Work out the finished part from the listing and answer in its coordinate system (mm). Face numbers are marked on the shaded views. A direction names the side the tool comes from. Round coordinates to 2 decimals unless told otherwise and drop trailing zeros. Loops run counter-clockwise (first coordinate to the right, second up) from the corner with the lowest first, then second, coordinate; pieces in that order, holes last. Notation, with made-up numbers: (12.5, 43.25) - (29.5, 43.25) arc R34 cw to (29.5, 73.25) - close; hole circle Ø11 at (69.25, 11.5). An arc over 180 degrees is marked (long way). Return JSON: item names as keys, results as strings.
from build123d import *

# Parameters (mm, degrees)
BOSS_EXTRUDE1_DEPTH = 6.2
BOSS_EXTRUDE2_DEPTH = 21
CHAMFER1_SIZE       = 5
CHAMFER1_SIZE2      = 28.356409098
CUT_EXTRUDE1_REACH  = 74.109
CHAMFER2_SIZE       = 1
CHAMFER2_SIZE2      = 9.514364454
CHAMFER3_SIZE       = 2
CUT_EXTRUDE2_REACH  = 79.092
CUT_EXTRUDE3_START  = -3.468867
CUT_EXTRUDE3_DEPTH  = 3.468867
BOSS_EXTRUDE3_DEPTH = 6.2
CUT_EXTRUDE4_REACH  = 79.092
CUT_EXTRUDE5_DEPTH  = 73.108598655
CUT_EXTRUDE6_REACH  = 74.109


with BuildPart() as part:
    # Sketch1 → Boss-Extrude1 (new body)
    with BuildSketch(Plane.XY):
        with BuildLine():
            Line((-28.3, 0), (0, 0))
            Line((0, 0), (0, 10))
            Line((0, 10), (-7.1, 10))
            ThreePointArc((-7.1, 10), (-14.171067812, 12.928932188), (-17.1, 20))
            Line((-17.1, 20), (-17.1, 51))
            Line((-17.1, 51), (-20.1, 51))
            Line((-20.1, 51), (-20.1, 6))
            Line((-20.1, 6), (-24.3, 6))
            Line((-24.3, 6), (-24.3, 50))
            Line((-24.3, 50), (-28.3, 50))
            Line((-28.3, 50), (-28.3, 0))
        make_face()
    extrude(amount=BOSS_EXTRUDE1_DEPTH)

    # Sketch2 → Boss-Extrude2 (add)
    with BuildSketch(Plane.XZ):
        Polygon((0, 6.2), (0, 10.4), (11, 10.4), (11, 42.4), (-24.1, 42.4), (-24.1, 10.4), (-13.1, 10.4), (-13.1, 6.2), align=None)
    extrude(amount=-BOSS_EXTRUDE2_DEPTH)

    # Chamfer1
    chamfer1_edges = [part.edges().sort_by_distance(p)[0] for p in [
        (-6.55, 0, 42.4),
    ]]
    chamfer1_side = [part.faces().sort_by_distance(p)[0] for p in [
        (-6.55, 10.5, 42.4),
    ]]
    chamfer(chamfer1_edges, length=CHAMFER1_SIZE, length2=CHAMFER1_SIZE2, reference=chamfer1_side[0])

    # Sketch3 → Cut-Extrude1 (cut, up to next)
    with BuildSketch(Plane(origin=(0, 0, 0), x_dir=(0, 0, -1), z_dir=(1, 0, 0)), mode=Mode.PRIVATE) as cut_extrude1_sk1:
        Polygon((-6.2, 10), (-7.6, 10), (-10.4, 21), (-6.2, 21), align=None)
    cut_extrude1_tool1 = extrude(cut_extrude1_sk1.sketch, amount=-CUT_EXTRUDE1_REACH, mode=Mode.PRIVATE) & part.part
    add(cut_extrude1_tool1.solids().sort_by_distance((0, 16.416667, 7.716667))[0], mode=Mode.SUBTRACT)

    # Chamfer2
    chamfer2_edges = [part.edges().sort_by_distance(p)[0] for p in [
        (11, 10.5, 10.4),
    ]]
    chamfer2_side = [part.faces().sort_by_distance(p)[0] for p in [
        (11, 11.541747932, 25.62778603),
    ]]
    chamfer(chamfer2_edges, length=CHAMFER2_SIZE, length2=CHAMFER2_SIZE2, reference=chamfer2_side[0])

    # Chamfer3
    chamfer3_edges = [part.edges().sort_by_distance(p)[0] for p in [
        (-24.1, 10.5, 10.4),
    ]]
    chamfer(chamfer3_edges, length=CHAMFER3_SIZE)

    # Sketch5 → Cut-Extrude2 (cut, up to next)
    with BuildSketch(Plane(origin=(11, 0, 0), x_dir=(0, 0, -1), z_dir=(1, 0, 0)), mode=Mode.PRIVATE) as cut_extrude2_sk1:
        Polygon((-42.4, 17.8), (-13.86886709, 5), (-10.966215349, -4.108657177), (-44.036924755, 0.937700744), align=None)
    cut_extrude2_tool1 = extrude(cut_extrude2_sk1.sketch, amount=-CUT_EXTRUDE2_REACH, mode=Mode.PRIVATE) & part.part
    add(cut_extrude2_tool1.solids().sort_by_distance((11, 5.258773, 29.627692))[0], mode=Mode.SUBTRACT)

    # Sketch6 → Cut-Extrude3 (cut)
    with BuildSketch(Plane(origin=(0, 0, 10.4), x_dir=(-1, 0, 0), z_dir=(0, 0, -1)).offset(CUT_EXTRUDE3_START)):
        Polygon((13.1, 0), (24.1, 5), (37.198342989, 5), (28.62602328, -4.522208447), (-13.825974113, -5.629287686), (-20.705007466, 5), (-11, 5), (0, 0), align=None)
    extrude(amount=CUT_EXTRUDE3_DEPTH, mode=Mode.SUBTRACT)

    # Sketch7 → Boss-Extrude3 (add)
    with BuildSketch(Plane.XY.offset(6.2)):
        with BuildLine():
            Line((-16.7, 50.6), (-15.7, 50.5))
            ThreePointArc((-15.7, 50.5), (-15.462165524, 50.365875857), (-15.4, 50.1))
            ThreePointArc((-15.4, 50.1), (-15.462165524, 49.834124143), (-15.7, 49.7))
            Line((-15.7, 49.7), (-16.7, 49.6))
            ThreePointArc((-16.7, 49.6), (-16.971392676, 49.471392676), (-17.1, 49.2))
            Line((-17.1, 49.2), (-17.1, 48.7))
            ThreePointArc((-17.1, 48.7), (-16.971392676, 48.428607324), (-16.7, 48.3))
            Line((-16.7, 48.3), (-15.7, 48.2))
            ThreePointArc((-15.7, 48.2), (-15.462165524, 48.065875857), (-15.4, 47.8))
            ThreePointArc((-15.4, 47.8), (-15.462165524, 47.534124143), (-15.7, 47.4))
            Line((-15.7, 47.4), (-16.7, 47.3))
            ThreePointArc((-16.7, 47.3), (-16.971392676, 47.171392676), (-17.1, 46.9))
            Line((-17.1, 46.9), (-17.1, 46.4))
            ThreePointArc((-17.1, 46.4), (-16.971392676, 46.128607324), (-16.7, 46))
            Line((-16.7, 46), (-15.7, 45.9))
            ThreePointArc((-15.7, 45.9), (-15.462165524, 45.765875857), (-15.4, 45.5))
            ThreePointArc((-15.4, 45.5), (-15.462165524, 45.234124143), (-15.7, 45.1))
            Line((-15.7, 45.1), (-16.7, 45))
            ThreePointArc((-16.7, 45), (-16.971392676, 44.871392676), (-17.1, 44.6))
            Line((-17.1, 44.6), (-17.1, 44.1))
            ThreePointArc((-17.1, 44.1), (-16.971392676, 43.828607324), (-16.7, 43.7))
            Line((-16.7, 43.7), (-15.7, 43.6))
            ThreePointArc((-15.7, 43.6), (-15.462165524, 43.465875857), (-15.4, 43.2))
            ThreePointArc((-15.4, 43.2), (-15.462165524, 42.934124143), (-15.7, 42.8))
            Line((-15.7, 42.8), (-16.7, 42.7))
            ThreePointArc((-16.7, 42.7), (-16.971392676, 42.571392676), (-17.1, 42.3))
            Line((-17.1, 42.3), (-17.1, 41.8))
            ThreePointArc((-17.1, 41.8), (-16.971392676, 41.528607324), (-16.7, 41.4))
            Line((-16.7, 41.4), (-15.7, 41.3))
            ThreePointArc((-15.7, 41.3), (-15.462165524, 41.165875857), (-15.4, 40.9))
            ThreePointArc((-15.4, 40.9), (-15.462165524, 40.634124143), (-15.7, 40.5))
            Line((-15.7, 40.5), (-16.7, 40.4))
            ThreePointArc((-16.7, 40.4), (-16.971392676, 40.271392676), (-17.1, 40))
            Line((-17.1, 40), (-17.1, 39.5))
            ThreePointArc((-17.1, 39.5), (-16.971392676, 39.228607324), (-16.7, 39.1))
            Line((-16.7, 39.1), (-15.7, 39))
            ThreePointArc((-15.7, 39), (-15.462165524, 38.865875857), (-15.4, 38.6))
            ThreePointArc((-15.4, 38.6), (-15.462165524, 38.334124143), (-15.7, 38.2))
            Line((-15.7, 38.2), (-16.7, 38.1))
            ThreePointArc((-16.7, 38.1), (-16.971392676, 37.971392676), (-17.1, 37.7))
            Line((-17.1, 37.7), (-17.1, 37.2))
            ThreePointArc((-17.1, 37.2), (-16.971392676, 36.928607324), (-16.7, 36.8))
            Line((-16.7, 36.8), (-15.7, 36.7))
            ThreePointArc((-15.7, 36.7), (-15.462165524, 36.565875857), (-15.4, 36.3))
            ThreePointArc((-15.4, 36.3), (-15.462165524, 36.034124143), (-15.7, 35.9))
            Line((-15.7, 35.9), (-16.7, 35.8))
            ThreePointArc((-16.7, 35.8), (-16.971392676, 35.671392676), (-17.1, 35.4))
            Line((-17.1, 35.4), (-17.1, 34.9))
            ThreePointArc((-17.1, 34.9), (-16.971392676, 34.628607324), (-16.7, 34.5))
            Line((-16.7, 34.5), (-15.7, 34.4))
            ThreePointArc((-15.7, 34.4), (-15.462165524, 34.265875857), (-15.4, 34))
            ThreePointArc((-15.4, 34), (-15.462165524, 33.734124143), (-15.7, 33.6))
            Line((-15.7, 33.6), (-16.7, 33.5))
            ThreePointArc((-16.7, 33.5), (-16.971392676, 33.371392676), (-17.1, 33.1))
            Line((-17.1, 33.1), (-17.1, 32.6))
            ThreePointArc((-17.1, 32.6), (-16.971392676, 32.328607324), (-16.7, 32.2))
            Line((-16.7, 32.2), (-15.7, 32.1))
            ThreePointArc((-15.7, 32.1), (-15.462165524, 31.965875857), (-15.4, 31.7))
            ThreePointArc((-15.4, 31.7), (-15.462165524, 31.434124143), (-15.7, 31.3))
            Line((-15.7, 31.3), (-16.7, 31.2))
            ThreePointArc((-16.7, 31.2), (-16.971392676, 31.071392676), (-17.1, 30.8))
            Line((-17.1, 30.8), (-17.1, 30.3))
            ThreePointArc((-17.1, 30.3), (-16.971392676, 30.028607324), (-16.7, 29.9))
            Line((-16.7, 29.9), (-15.7, 29.8))
            ThreePointArc((-15.7, 29.8), (-15.462165524, 29.665875857), (-15.4, 29.4))
            ThreePointArc((-15.4, 29.4), (-15.462165524, 29.134124143), (-15.7, 29))
            Line((-15.7, 29), (-16.7, 28.9))
            ThreePointArc((-16.7, 28.9), (-16.971392676, 28.771392676), (-17.1, 28.5))
            Line((-17.1, 28.5), (-17.1, 28))
            ThreePointArc((-17.1, 28), (-16.971392676, 27.728607324), (-16.7, 27.6))
            Line((-16.7, 27.6), (-15.7, 27.5))
            ThreePointArc((-15.7, 27.5), (-15.462165524, 27.365875857), (-15.4, 27.1))
            ThreePointArc((-15.4, 27.1), (-15.462165524, 26.834124143), (-15.7, 26.7))
            Line((-15.7, 26.7), (-16.7, 26.6))
            ThreePointArc((-16.7, 26.6), (-16.971392676, 26.471392676), (-17.1, 26.2))
            Line((-17.1, 26.2), (-17.1, 25.7))
            ThreePointArc((-17.1, 25.7), (-16.971392676, 25.428607324), (-16.7, 25.3))
            Line((-16.7, 25.3), (-15.7, 25.2))
            ThreePointArc((-15.7, 25.2), (-15.462165524, 25.065875857), (-15.4, 24.8))
            ThreePointArc((-15.4, 24.8), (-15.462165524, 24.534124143), (-15.7, 24.4))
            Line((-15.7, 24.4), (-16.7, 24.3))
            ThreePointArc((-16.7, 24.3), (-16.971392676, 24.171392676), (-17.1, 23.9))
            Line((-17.1, 23.9), (-17.1, 23.4))
            ThreePointArc((-17.1, 23.4), (-16.971392676, 23.128607324), (-16.7, 23))
            Line((-16.7, 23), (-15.7, 22.9))
            ThreePointArc((-15.7, 22.9), (-15.462165524, 22.765875857), (-15.4, 22.5))
            ThreePointArc((-15.4, 22.5), (-15.462165524, 22.234124143), (-15.7, 22.1))
            Line((-15.7, 22.1), (-16.7, 22))
            ThreePointArc((-16.7, 22), (-16.971392676, 21.871392676), (-17.1, 21.6))
            Line((-17.1, 21.6), (-17.1, 21.1))
            ThreePointArc((-17.1, 21.1), (-16.971392676, 20.828607324), (-16.7, 20.7))
            Line((-16.7, 20.7), (-15.7, 20.6))
            ThreePointArc((-15.7, 20.6), (-15.462165524, 20.465875857), (-15.4, 20.2))
            ThreePointArc((-15.4, 20.2), (-15.462165524, 19.934124143), (-15.7, 19.8))
            Line((-15.7, 19.8), (-16.7, 19.7))
            ThreePointArc((-16.7, 19.7), (-16.971392676, 19.571392676), (-17.1, 19.3))
            Line((-17.1, 19.3), (-17.1, 18.8))
            Line((-17.1, 18.8), (-18.685, 49.2))
            Line((-18.685, 49.2), (-17.1, 51))
            ThreePointArc((-17.1, 51), (-16.971392676, 50.728607324), (-16.7, 50.6))
        make_face()
    extrude(amount=-BOSS_EXTRUDE3_DEPTH)

    # Sketch8 → Cut-Extrude4 (cut, up to next)
    with BuildSketch(Plane(origin=(11, 0, 0), x_dir=(0, 0, -1), z_dir=(1, 0, 0)), mode=Mode.PRIVATE) as cut_extrude4_sk1:
        Polygon((-35.4, 21), (-27.4, 17), (-19.4, 21), align=None)
    cut_extrude4_tool1 = extrude(cut_extrude4_sk1.sketch, amount=-CUT_EXTRUDE4_REACH, mode=Mode.PRIVATE) & part.part
    add(cut_extrude4_tool1.solids().sort_by_distance((11, 19.666667, 27.4))[0], mode=Mode.SUBTRACT)

    # Sketch10 → Cut-Extrude5 (cut, through all)
    with BuildSketch(Plane.XY.offset(42.4)):
        Polygon((-11.55, 21), (-6.55, 19), (-1.55, 21), align=None)
    extrude(amount=-CUT_EXTRUDE5_DEPTH, mode=Mode.SUBTRACT)

    # Sketch11 → Cut-Extrude6 (cut, up to next)
    with BuildSketch(Plane(origin=(0, 0, 0), x_dir=(-1, 0, 0), z_dir=(0, 0, -1)), mode=Mode.PRIVATE) as cut_extrude6_sk1:
        Polygon((24.3, 23.549969474), (24.6, 5.974018531), (19.8, 5.974018531), (20.1, 30.243837205), align=None)
    cut_extrude6_tool1 = extrude(cut_extrude6_sk1.sketch, amount=-CUT_EXTRUDE6_REACH, mode=Mode.PRIVATE) & part.part
    add(cut_extrude6_tool1.solids().sort_by_distance((-22.072028, 16.298165, 0))[0], mode=Mode.SUBTRACT)


solid = part.part
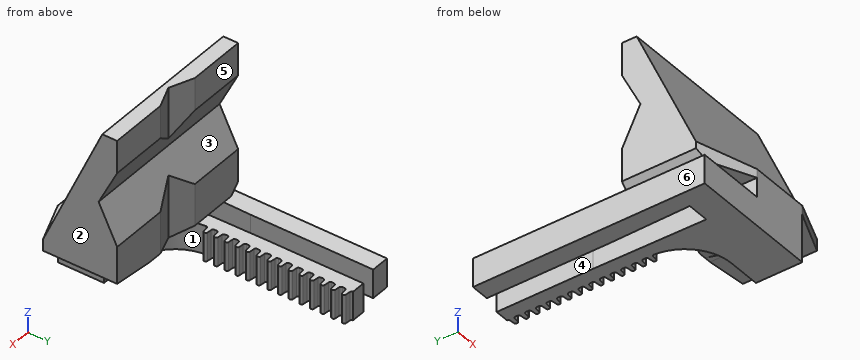
1) Find the intervals of material crossed by L1, parallel to X at y = 13.5, z = 32; L2, parallel to Z at x = -16, y = 32; L3, parallel to Y at x = -22, z = 2, in increasing order.
Verdict:
{"L1": "x = -24.1 to 11", "L2": "z = 0 to 6.2", "L3": "y = 0 to 5.97"}
2) Section A-A (y = 13) is taken. Give the vertices of the cut face in (x, z), and give its area (3 significant figures).
Verdict:
{"outline": "(-28.3, 0) - (-24.48, 0) - (-24.48, 6.2) - (-28.3, 6.2) - close; (-24.1, 12.4) - (-22.1, 10.4) - (-13.1, 10.4) - (-13.1, 8.36) - (0, 8.36) - (0, 10.4) - (1.49, 10.4) - (11, 11.4) - (11, 31.7) - (-24.1, 31.7) - close; (-19.89, 0) - (-14.24, 0) - (-14.24, 6.2) - (-19.89, 6.2) - close", "area": "826 mm2"}
3) Determine the mould class of the marked faces 1, 2 and 3 for opening direction Y: pulls with the +Y half, pulls with the -Y half, needs draft (parallel to the pull), parting line crosses it, or undercut.
Verdict:
{"face 1": "undercut", "face 2": "needs draft", "face 3": "pulls with the +Y half"}
4) Section C-C (x = -21) is taken. Give the vertices of the cut face in (y, z).
Verdict:
{"outline": "(0, 0) - (5.97, 0) - (5.97, 6.2) - (0, 6.2) - close; (3.59, 10.4) - (21, 10.4) - (21, 19.4) - (17, 27.4) - (21, 35.4) - (21, 42.4) - (17.8, 42.4) - (5, 13.87) - (3.59, 13.42) - close"}
5) Section B-B (z = 38) is taken. Give the vertices of the cut face in (x, y).
Verdict:
{"outline": "(-24.1, 15.83) - (11, 15.83) - (11, 21) - (-1.55, 21) - (-6.55, 19) - (-11.55, 21) - (-24.1, 21) - close"}
6) Section D-D (z = 17) is taken. Give the vertices of the cut face in (x, y), and give its area (3 significant figures).
Verdict:
{"outline": "(-24.1, 6.4) - (11, 6.4) - (11, 21) - (-1.55, 21) - (-6.55, 19) - (-11.55, 21) - (-24.1, 21) - close", "area": "502 mm2"}
7) Flat-ended cylindrical pins translate along their axes: pin 1 (8 mm diameter, centred on x = -19, y = 6.5, fed in from +Z); pin 2 (0.6 mm diameter, centred on y = 49, z = 2.5, fed in from +X); pin 3 (3 mm diameter, centred on x = -27, z = 1.5, fed in from +Y); pin 4 (4 mm diameter, centred on x = 3, z = 8, fed in from -Y). Find the tip coordinate at first contact, or state that the pin passes through.
Verdict:
{"pin 1": "stops at z = 26.13", "pin 2": "stops at x = -17.08", "pin 3": "stops at y = 50", "pin 4": "passes through"}
8) A tool of negligible diameter and unlimited length cuts with its end or side. For the marked faces 4, 5 and 6, from which of +Z, -Z, +X, -X, +Y, -Y can it reach the whole face along a straight path? Write none if from no direction.
Verdict:
{"face 4": "+Z, -Z, +Y", "face 5": "+Z, +X, -X, +Y", "face 6": "+Z, -Z, -X, +Y, -Y"}
